The listing builds one solid part. Answer for the finished solid, in the listing's coordinates (mm). A direction names the side the tool comes from. Give positions to 0.01 mm unless a question says otherwise; leave off trailing zeros. Write each loop counter-clockwise with the first axis right and the second up, starting at its lowest first coordinate (ties: lowest second). Pieces come first, ordered by that corner, then holes. Notation, with made-up numbers: (-0.75, 44.25) - (4.25, 44.25) arc R18 cw to (4.25, 72.25) - close; hole circle Ø8 at (87, -8). An arc over 180 degrees is marked (long way). One line per item, written item: value. Start each with the question number.
from build123d import *

# Parameters (mm, degrees)
SKETCH1_W               = 152.4
SKETCH1_H               = 127
BOSS_EXTRUDE1_DEPTH     = 2.3622
FILLET1_R               = 2.54
SKETCH9_R               = 4.15
CUT_EXTRUDE8_DEPTH      = 100.218294628
CUT_EXTRUDE11_DEPTH     = 100.218294628
CUT_EXTRUDE12_DEPTH     = 100.218294628
SKETCH16_R              = 4.15
CUT_EXTRUDE14_DEPTH     = 100.218294628
SKETCH17_R              = 2.7305
CUT_EXTRUDE16_DEPTH     = 100.218294628
MIRROR7_COPY_1_SKETCH_R = 2.7305
MIRROR7_COPY_1_DEPTH    = 100.218294628
SKETCH26_W              = 10.16
SKETCH26_H              = 12.7
CUT_EXTRUDE26_DEPTH     = 100.218294628
SKETCH27_R              = 4.15
CUT_EXTRUDE27_DEPTH     = 100.218294628
SKETCH29_R              = 4.15
CUT_EXTRUDE28_DEPTH     = 100.218294628
SKETCH30_R              = 4.15
CUT_EXTRUDE29_DEPTH     = 100.218294628
SKETCH31_R              = 4.15
CUT_EXTRUDE30_DEPTH     = 100.218294628
CUT_EXTRUDE31_DEPTH     = 0.79375
SKETCH33_W              = 1.5875
SKETCH33_H              = 1.5875
CUT_EXTRUDE32_DEPTH     = 0.79375
SKETCH34_W              = 24.632574661
SKETCH34_H              = 37.675
SKETCH34_W_2            = 21.457574661
SKETCH34_H_2            = 34.5
CUT_EXTRUDE33_DEPTH     = 0.79375
CUT_EXTRUDE34_START     = -0.79375
CUT_EXTRUDE34_DEPTH     = 0.79375


with BuildPart() as part:
    # Sketch1 → Boss-Extrude1 (new body)
    with BuildSketch(Plane(origin=(0, 0, 0), x_dir=(1, 0, 0), z_dir=(0, 1, 0))):
        Rectangle(SKETCH1_W, SKETCH1_H)
    extrude(amount=BOSS_EXTRUDE1_DEPTH)

    # Fillet1
    fillet1_edges = [part.edges().sort_by_distance(p)[0] for p in [
        (76.2, 1.1811, 63.5),
        (-76.2, 1.1811, 63.5),
        (-76.2, 1.1811, -63.5),
        (76.2, 1.1811, -63.5),
    ]]
    fillet(fillet1_edges, radius=FILLET1_R)

    # Sketch9 → Cut-Extrude8 (cut, through all)
    with BuildSketch(Plane.XZ):
        with Locations(Location((60.8584, 27.94, 0), (0, 0, 270))):
            Circle(SKETCH9_R)
        with Locations(Location((60.8584, -2.54, 0), (0, 0, 270))):
            Circle(SKETCH9_R)
    extrude(amount=-CUT_EXTRUDE8_DEPTH, mode=Mode.SUBTRACT)

    # Sketch12 → Cut-Extrude11 (cut, through all)
    with BuildSketch(Plane.XZ):
        with BuildLine():
            Line((-3.81, 59.465627528), (3.81, 59.465627528))
            ThreePointArc((3.81, 59.465627528), (8.387405636, 54.888221892), (3.81, 50.310816255))
            Line((3.81, 50.310816255), (-3.81, 50.310816255))
            ThreePointArc((-3.81, 50.310816255), (-8.387405636, 54.888221892), (-3.81, 59.465627528))
        make_face()
    cut_extrude11 = extrude(amount=-CUT_EXTRUDE11_DEPTH, mode=Mode.SUBTRACT)

    # Mirror3: Cut-Extrude11 across plane
    add(cut_extrude11.mirror(Plane.XY), mode=Mode.SUBTRACT)

    # Sketch13 → Cut-Extrude12 (cut, through all)
    with BuildSketch(Plane(origin=(0, 0, 0), x_dir=(-1, 0, 0), z_dir=(0, -1, 0))):
        with BuildLine():
            Line((60.052874771, -48.26), (60.052874771, -55.88))
            ThreePointArc((60.052874771, -55.88), (55.88, -60.052874771), (51.707125229, -55.88))
            Line((51.707125229, -55.88), (51.707125229, -48.26))
            ThreePointArc((51.707125229, -48.26), (55.88, -44.087125229), (60.052874771, -48.26))
        make_face()
    extrude(amount=-CUT_EXTRUDE12_DEPTH, mode=Mode.SUBTRACT)

    # Sketch16 → Cut-Extrude14 (cut, through all)
    with BuildSketch(Plane(origin=(0, 0, 0), x_dir=(-1, 0, 0), z_dir=(0, -1, 0))):
        with Locations(Location((-69.599893995, 19.704320306, 0), (0, 0, 90))):
            Circle(SKETCH16_R)
        with Locations(Location((-46.522565834, 32.264238523, 0), (0, 0, 90))):
            Circle(SKETCH16_R)
    extrude(amount=-CUT_EXTRUDE14_DEPTH, mode=Mode.SUBTRACT)

    # Sketch17 → Cut-Extrude16 (cut, through all)
    with BuildSketch(Plane.XZ):
        with Locations(Location((71.794813785, 59.510435834, 0), (0, 0, 270))):
            Circle(SKETCH17_R)
    cut_extrude16 = extrude(amount=-CUT_EXTRUDE16_DEPTH, mode=Mode.SUBTRACT)

    # Mirror6: Cut-Extrude16 across plane
    add(cut_extrude16.mirror(Plane(origin=(0, 0, 0), x_dir=(0, 0, 1), z_dir=(1, 0, 0))), mode=Mode.SUBTRACT)

    # Mirror7: Cut-Extrude16 across plane
    add(cut_extrude16.mirror(Plane.XY), mode=Mode.SUBTRACT)

    # Mirror7 copy 1 sketch → Mirror7 copy 1 (cut, through all)
    with BuildSketch(Plane(origin=(0, 0, 0), x_dir=(-1, 0, 0), z_dir=(0, -1, 0))):
        with Locations(Location((71.794813785, 59.510435834, 0), (0, 0, 270))):
            Circle(MIRROR7_COPY_1_SKETCH_R)
    extrude(amount=-MIRROR7_COPY_1_DEPTH, mode=Mode.SUBTRACT)

    # Sketch26 → Cut-Extrude26 (cut, through all)
    with BuildSketch(Plane(origin=(0, 2.3622, 0), x_dir=(1, 0, 0), z_dir=(0, 1, 0))):
        with Locations((18.964621702, 0)):
            Rectangle(SKETCH26_W, SKETCH26_H)
    extrude(amount=-CUT_EXTRUDE26_DEPTH, mode=Mode.SUBTRACT)

    # Sketch27 → Cut-Extrude27 (cut, through all)
    with BuildSketch(Plane.XZ):
        with Locations(Location((-59.831398438, 33.060447312, 0), (0, 0, 270))):
            Circle(SKETCH27_R)
        with Locations(Location((-50.09170874, -30.48, 0), (0, 0, 270))):
            Circle(SKETCH27_R)
    extrude(amount=-CUT_EXTRUDE27_DEPTH, mode=Mode.SUBTRACT)

    # Sketch29 → Cut-Extrude28 (cut, through all)
    with BuildSketch(Plane(origin=(0, 2.3622, 0), x_dir=(1, 0, 0), z_dir=(0, 1, 0))):
        with Locations(Location((18.964621702, 19.681240592, 0), (0, 0, 270))):
            Circle(SKETCH29_R)
        with Locations(Location((18.964621702, -19.681240592, 0), (0, 0, 270))):
            Circle(SKETCH29_R)
    extrude(amount=-CUT_EXTRUDE28_DEPTH, mode=Mode.SUBTRACT)

    # Sketch30 → Cut-Extrude29 (cut, through all)
    with BuildSketch(Plane(origin=(0, 2.3622, 0), x_dir=(1, 0, 0), z_dir=(0, 1, 0))):
        with Locations(Location((69.803274088, -49.53, 0), (0, 0, 270))):
            Circle(SKETCH30_R)
        with Locations(Location((30.63517528, -49.53, 0), (0, 0, 270))):
            Circle(SKETCH30_R)
    cut_extrude29 = extrude(amount=-CUT_EXTRUDE29_DEPTH, mode=Mode.SUBTRACT)

    # Mirror8: Cut-Extrude29 across plane
    add(cut_extrude29.mirror(Plane.XY), mode=Mode.SUBTRACT)

    # Sketch31 → Cut-Extrude30 (cut, through all)
    with BuildSketch(Plane(origin=(0, 2.3622, 0), x_dir=(1, 0, 0), z_dir=(0, 1, 0))):
        with Locations(Location((-63.894835235, -12.79551579, 0), (0, 0, 270))):
            Circle(SKETCH31_R)
        with Locations(Location((-63.894835235, 13.549600091, 0), (0, 0, 270))):
            Circle(SKETCH31_R)
    extrude(amount=-CUT_EXTRUDE30_DEPTH, mode=Mode.SUBTRACT)

    # Sketch32 → Cut-Extrude31 (cut)
    with BuildSketch(Plane(origin=(0, 2.3622, 0), x_dir=(1, 0, 0), z_dir=(0, 1, 0))):
        Polygon((-66.467594082, 36.762943521), (-56.233474354, 36.762943521), (-56.233474354, 36.855969312), (-43.767784695, 36.855969312), (-43.767784695, 36.762943521), (-43.689716795, 36.762943521), (-43.689716795, 17.806129276), (-42.180284695, 17.806129276), (-42.180284695, 38.350443521), (-68.055094082, 38.350443521), (-68.055094082, 17.806129276), (-66.467594082, 17.806129276), align=None)
        Polygon((-43.533580996, -39.436416624), (-66.155322484, -39.436416624), (-66.155322484, -20.293550797), (-67.742822484, -20.293550797), (-67.742822484, -41.023916624), (-41.946080996, -41.023916624), (-41.946080996, -20.293550797), (-43.533580996, -20.293550797), align=None)
    extrude(amount=-CUT_EXTRUDE31_DEPTH, mode=Mode.SUBTRACT)

    # Sketch33 → Cut-Extrude32 (cut)
    with BuildSketch(Plane(origin=(0, 2.3622, 0), x_dir=(1, 0, 0), z_dir=(0, 1, 0))):
        Polygon((51.297781708, 11.125983721), (49.710281708, 11.125983721), (49.710281708, -39.6875), (76.2, -39.6875), (76.2, -38.1), (51.297781708, -38.1), align=None)
        Polygon((76.184917735, 12.713483721), (51.297781708, 12.713483721), (51.297781708, 11.125983721), (76.2, 11.125983721), (76.2, 14.063999978), (76.184917735, 14.063999978), align=None)
        with Locations((50.504031708, 11.919733721)):
            Rectangle(SKETCH33_W, SKETCH33_H)
        Polygon((49.710281708, 12.713483721), (40.669704347, 12.713483721), (40.669704347, 38.10435014), (76.184917735, 38.10435014), (76.184917735, 14.063999978), (76.2, 14.063999978), (76.2, 39.69185014), (39.082204347, 39.69185014), (39.082204347, 11.125983721), (49.710281708, 11.125983721), align=None)
    extrude(amount=-CUT_EXTRUDE32_DEPTH, mode=Mode.SUBTRACT)

    # Sketch34 → Cut-Extrude33 (cut)
    with BuildSketch(Plane.XZ):
        with Locations((-63.883712669, -0.37704215)):
            Rectangle(SKETCH34_W, SKETCH34_H)
        with Locations((-63.88371267, -0.37704215)):
            Rectangle(SKETCH34_W_2, SKETCH34_H_2, mode=Mode.SUBTRACT)
    extrude(amount=-CUT_EXTRUDE33_DEPTH, mode=Mode.SUBTRACT)

    # Sketch36 → Cut-Extrude34 (cut)
    with BuildSketch(Plane.XZ.offset(CUT_EXTRUDE34_START)):
        with BuildLine():
            Line((75.27317528, 44.45), (26.57117528, 44.45))
            Line((26.57117528, 44.45), (26.57117528, 48.689521566))
            ThreePointArc((26.57117528, 48.689521566), (26.48517528, 49.53), (26.57117528, 50.370478434))
            Line((26.57117528, 50.370478434), (26.57117528, 54.61))
            Line((26.57117528, 54.61), (75.27317528, 54.61))
            Line((75.27317528, 54.61), (75.27317528, 56.1975))
            Line((75.27317528, 56.1975), (24.98367528, 56.1975))
            Line((24.98367528, 56.1975), (24.98367528, 42.8625))
            Line((24.98367528, 42.8625), (75.27317528, 42.8625))
            Line((75.27317528, 42.8625), (75.27317528, 44.45))
        make_face()
    cut_extrude34 = extrude(amount=CUT_EXTRUDE34_DEPTH, mode=Mode.SUBTRACT)

    # Mirror9: Cut-Extrude34 across plane
    add(cut_extrude34.mirror(Plane.XY), mode=Mode.SUBTRACT)


solid = part.part
Item 1: Find section C-C on z = -30.48. Give the number of separate pieces and of enclosed holes in the cut face, plus the area to 3 significant figures.
Item 2: Find section B-B on z = 27. Determine the outline of the cut face in (x, y), plus the area to 3 significant figures.
Item 3: For faces 1 (the flat face through (58, 2.362, -26)), 2 (the cylindrical face through (-55.97, 1.16, 60.05)), determine the directions among +Z, -Z, +X, -X, +Y, -Y from which every point of the face is accessible in a straight line to the end or side of a thin tool.
Item 4: The mould has two halves that part along Z. Classify faces 3 (the flat face through (-57, 1.568, -37)), 4 (the cylindrical face through (73.303, 1.198, 51.761)), 5 (the flat face through (-1, 2.362, -1)): +Z half, -Z half, draft (parallel to the pull), parting line (faces both ways), or undercut.
Item 5: Straight lines are drawn through the part: line 1 along X through (y, z) = (1.25, -49.53); line 2 along Z through (x, y) = (-61.5, 1.2); line 3 along Z through (x, y) = (49.5, 1.8). For each, find the intervals that lie inside material, in ascending order.
Item 6: Find section A-A on z = -2.54. Determine the outline of the cut face in (x, y).
Values:
1. separate pieces: 3
1. enclosed holes: 0
1. area: 319 mm^2
2. outline: (-76.2, 0) - (56.82, 0) - (56.82, 2.36) - (51.3, 2.36) - (51.3, 1.57) - (49.71, 1.57) - (49.71, 2.36) - (-41.95, 2.36) - (-41.95, 1.57) - (-43.53, 1.57) - (-43.53, 2.36) - (-66.16, 2.36) - (-66.16, 1.57) - (-67.74, 1.57) - (-67.74, 2.36) - (-76.2, 2.36) - close; (64.9, 0) - (76.2, 0) - (76.2, 2.36) - (64.9, 2.36) - close
2. area: 337 mm^2
3. face 1: +Z, -Z, +X, -X, +Y
3. face 2: +Y, -Y
4. face 3: undercut
4. face 4: undercut
4. face 5: draft
5. line 1: -76.2 to 26.49, 34.79 to 65.65, 73.95 to 76.2
5. line 2: -63.5 to -16.94, -10.16 to 9.41, 16.18 to 29.26, 36.86 to 63.5
5. line 3: -63.5 to -39.69, -38.1 to -35.16, -29.37 to -12.71, -11.13 to 63.5
6. outline: (-76.2, 0.79) - (-74.61, 0.79) - (-74.61, 0) - (-53.15, 0) - (-53.15, 0.79) - (-51.57, 0.79) - (-51.57, 0) - (13.88, 0) - (13.88, 2.36) - (-76.2, 2.36) - close; (24.04, 0) - (56.71, 0) - (56.71, 2.36) - (51.3, 2.36) - (51.3, 1.57) - (49.71, 1.57) - (49.71, 2.36) - (24.04, 2.36) - close; (65.01, 0) - (76.2, 0) - (76.2, 2.36) - (65.01, 2.36) - close
